Geometry: final body of the model. Coordinates: model frame, mm. A direction names the side the tool comes from. Coordinates: 2 decimals unless noted, no trailing zeros. Order: outer loops, then holes, each group sorted by start corner. A loop starts at its lowest first (then second) coordinate and runs counter-clockwise, first axis right, second up. Notation, with made-up numbers: M 81.25,43 L 131.25,43 A19 cw 131.25,76 Z; hole C -9.75,0.25 d8. An arc over 180 degrees is marked long. Use CSV: the item, a comma, the result in double quotes. Start each with the question number.
1. Section query A-A on z = 0.5. Return the cut outline in (x, y), and give its area (4 significant figures).
2. First-contact query: P1, Ø10, axis at x = 7, y = 11.5, coming from the -Z side; P2, Ø10, axis at y = 7, z = -4.5, coming from the -X side; P3, Ø1.5, axis at y = 18, z = 2.5, coming from the +X side. Flat tips, straight axial feed; report the tip coordinate or a pass-through.
3. Section query B-B on x = 8. Return the cut outline in (y, z).
4. Section query C-C on y = 12.5. Return the cut outline in (x, z), and give its area (3 significant figures).
5. Material intervals for line 1 (Y direction, x = 13, z = -7.5); line 2 (X direction, y = 7.5, z = 5.25); line 3 (Z direction, x = -20, y = 16), sorted ascending.
6. Pull-direction query (X, two-part tool) for faces 6 (the flat face through (-24, 20.5, 0.2)), 7 (the flat face through (-0.3, 20.5, 14.5)), 8 (the flat face through (0, 20.9, 0)); classes: pulls with the +X half, pulls with the -X half, needs draft (parallel to the pull), parting line crosses it, or undercut.
7. Set-up query: faces 1 (the flat face through (-2, 21, 14)), 2 (the flat face through (0, 10, -13)), 3 (the flat face through (22.5, 10, 0)), 4 (the flat face through (-22.5, 10, 0)), 5 (the flat face through (0, 10, 13)). Return all of +Z, -Z, +X, -X, +Y, -Y with unobstructed straight access to the full face (end or side cutting, diameter ignored); none if empty.
from build123d import *

# Parameters (mm, degrees)
SKETCH_1_W          = 45
SKETCH_1_H          = 26
EXTRUDE_4_DEPTH     = 20
SKETCH_3_W          = 48
SKETCH_3_H          = 29
EXTRUDE_5_DEPTH     = 1
SKETCH_4_W          = 45
SKETCH_4_H          = 26
CUT_EXTRUDE_1_DEPTH = 0.1


with BuildPart() as part:
    # 草图1 → 凸台-拉伸4 (new body)
    with BuildSketch(Plane(origin=(0, 0, 0), x_dir=(1, 0, 0), z_dir=(0, 1, 0))):
        Rectangle(SKETCH_1_W, SKETCH_1_H)
    extrude(amount=EXTRUDE_4_DEPTH)

    # 草图3 → 凸台-拉伸5 (add)
    with BuildSketch(Plane(origin=(0, 20, 0), x_dir=(1, 0, 0), z_dir=(0, 1, 0))):
        Rectangle(SKETCH_3_W, SKETCH_3_H)
    extrude(amount=EXTRUDE_5_DEPTH)

    # 草图4 → 切除-拉伸1 (cut)
    with BuildSketch(Plane(origin=(0, 21, 0), x_dir=(1, 0, 0), z_dir=(0, 1, 0))):
        Rectangle(SKETCH_4_W, SKETCH_4_H)
    extrude(amount=-CUT_EXTRUDE_1_DEPTH, mode=Mode.SUBTRACT)


solid = part.part
Results list:
1,outline,"M -24,20 L -22.5,20 L -22.5,0 L 22.5,0 L 22.5,20 L 24,20 L 24,21 L 22.5,21 L 22.5,20.9 L -22.5,20.9 L -22.5,21 L -24,21 Z"
1,area,"943.5 mm²"
2,P1,"stops at z = -13"
2,P2,"stops at x = -22.5"
2,P3,"stops at x = 22.5"
3,outline,"M 0,-13 L 20,-13 L 20,-14.5 L 21,-14.5 L 21,-13 L 20.9,-13 L 20.9,13 L 21,13 L 21,14.5 L 20,14.5 L 20,13 L 0,13 Z"
4,outline,"M -22.5,-13 L 22.5,-13 L 22.5,13 L -22.5,13 Z"
4,area,"1,170 mm²"
5,line 1,"y = 0 to 20.9"
5,line 2,"x = -22.5 to 22.5"
5,line 3,"z = -13 to 13"
6,face 6,"pulls with the -X half"
6,face 7,"needs draft"
6,face 8,"undercut"
7,face 1,"+Z, -Z, +X, -X, +Y"
7,face 2,"-Z, +X, -X, -Y"
7,face 3,"+Z, -Z, +X, -Y"
7,face 4,"+Z, -Z, -X, -Y"
7,face 5,"+Z, +X, -X, -Y"
